For this review, take the finished solid that the model builds, in its own axes (mm). Face numbers are marked on the shaded views. A direction names the side the tool comes from. Round coordinates to 2 decimals unless told otherwise and drop trailing zeros. Loops run counter-clockwise (first coordinate to the right, second up) from the corner with the lowest first, then second, coordinate; pieces in that order, holes last.
1) Tool access review of the marked faces 1 and 2: name each direction out of +Z, -Z, +X, -X, +Y, -Y from which nothing blocks a thin tool from reaching the whole face with its end or side.
2) Take a section at B-B (x = 21). State the section outline as (y, z) points.
3) Take a section at A-A (y = 0). State the section outline as (x, z) points, then the cut area to 3 significant figures.
4) Wall thickness on L1, parallel to X at y = -4.25, z = 3; L2, parallel to Y at x = 46, z = -3; L3, parallel to X at y = -5, z = -5.75: over which ranges is each line inside the solid? List them lowest first.
5) Insertion check: pin 1 (1.5 mm diameter, centred on x = 38.5, z = 4.5, fed in from +Y); pin 2 (4 mm diameter, centred on x = 17, y = -6, fed in from +Z); pin 3 (8 mm diameter, centred on x = 25.5, y = 0.5, fed in from +Z). Each pin has a flat end and moves straight along its axis. Give the tip position at first contact, or say it passes through.
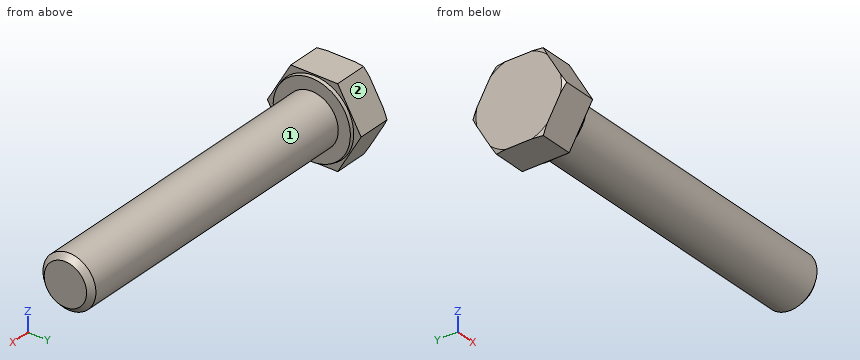
```python
from build123d import *

# Parameters (mm, degrees)
SKETCH_2_OUTSIDE_W  = 34.038
SKETCH_2_OUTSIDE_H  = 34.038
CUT_EXTRUDE_1_DEPTH = 69.335915886
CHAMFER_1_SIZE      = 1


with BuildPart() as part:
    # Эскиз1 → Повернуть1 (revolve)
    with BuildSketch(Plane.XY, mode=Mode.PRIVATE) as revolve_1_sk:
        Polygon((-6.58, 0), (-6.58, 8.85), (0, 8.85), (0, 7.448974596), (0.6, 7.288205081), (0.6, 5), (60.6, 5), (60.6, 0), align=None)
    revolve(revolve_1_sk.sketch.rotate(Axis((-1000, 0, 0), (1, 0, 0)), 90), axis=Axis((-1000, 0, 0), (1, 0, 0)))

    # Эскиз2 outside → Вырез-Вытянуть1 (cut, through all)
    with BuildSketch(Plane.ZY.offset(6.58)):
        Rectangle(SKETCH_2_OUTSIDE_W, SKETCH_2_OUTSIDE_H)
        Polygon((0, -8.85), (7.664324823, -4.425), (7.664324823, 4.425), (0, 8.85), (-7.664324823, 4.425), (-7.664324823, -4.425), align=None, mode=Mode.SUBTRACT)
    extrude(amount=-CUT_EXTRUDE_1_DEPTH, mode=Mode.SUBTRACT)

    # Эскиз4 → Вырез-Повернуть1 (revolve, cut)
    with BuildSketch(Plane.XY):
        Polygon((-6.58, 8.075), (-6.297923068, 8.85), (-6.58, 8.85), align=None)
    revolve(axis=Axis((-1000, 0, 0), (1, 0, 0)), mode=Mode.SUBTRACT)

    # Фаска1
    chamfer_1_edges = [part.edges().sort_by_distance(p)[0] for p in [
        (60.6, 0, -5),
    ]]
    chamfer(chamfer_1_edges, length=CHAMFER_1_SIZE)


solid = part.part
```
Response:
1. face 1: +X
1. face 2: +Z, +X, -X, +Y
2. outline: circle Ø10 at (0, 0)
3. outline: (-6.58, -7.66) - (0, -7.66) - (0, -7.45) - (0.6, -7.29) - (0.6, -5) - (59.6, -5) - (60.6, -4) - (60.6, 4) - (59.6, 5) - (0.6, 5) - (0.6, 7.29) - (0, 7.45) - (0, 7.66) - (-6.58, 7.66) - close
3. area: 709 mm2
4. L1: x = -6.58 to 0.6
4. L2: y = -4 to 4
4. L3: x = -6.58 to 0
5. pin 1: stops at y = 3.31
5. pin 2: stops at z = 3
5. pin 3: stops at z = 5
